Geometry check sheet. Reference: the model listing, model coordinates, mm. Face numbers are marked on the shaded views. A direction names the side the tool comes from. Give positions to 0.01 mm unless a question says otherwise; leave off trailing zeros. Order: outer loops, then holes, each group sorted by start corner. A loop starts at its lowest first (then second) coordinate and runs counter-clockwise, first axis right, second up. Notation, with made-up numbers: M 4,79 L 50,79 A15 cw 50,83 Z; hole C 28.5,73 d4. An arc over 180 degrees is marked long. Answer as CSV lines item,"result".
from build123d import *

# Parameters (mm, degrees)
ESQUISSE1_W             = 18
ESQUISSE1_H             = 34
BOSS_EXTRU_1_DEPTH      = 25
ESQUISSE2_R             = 3
ESQUISSE2_W             = 15
ESQUISSE2_H             = 24
ENL_V_MAT_EXTRU_1_DEPTH = 26
ESQUISSE3_R             = 3
ENL_V_MAT_EXTRU_2_DEPTH = 4
ESQUISSE4_R             = 4
ENL_V_MAT_EXTRU_3_DEPTH = 19


with BuildPart() as part:
    # Esquisse1 → Boss.-Extru.1 (new body)
    with BuildSketch(Plane.XY):
        with Locations((9, -17)):
            Rectangle(ESQUISSE1_W, ESQUISSE1_H)
    extrude(amount=BOSS_EXTRU_1_DEPTH)

    # Esquisse2 → Enlèv. mat.-Extru.1 (cut, through all)
    with BuildSketch(Plane.XY.offset(25)):
        with Locations((8, -29)):
            Circle(ESQUISSE2_R)
        with Locations((7.5, -12)):
            Rectangle(ESQUISSE2_W, ESQUISSE2_H)
    extrude(amount=-ENL_V_MAT_EXTRU_1_DEPTH, mode=Mode.SUBTRACT)

    # Esquisse3 → Enlèv. mat.-Extru.2 (cut)
    with BuildSketch(Plane(origin=(18, 0, 0), x_dir=(0, 0, -1), z_dir=(1, 0, 0))):
        with Locations((-12.5, -29)):
            Circle(ESQUISSE3_R)
    extrude(amount=-ENL_V_MAT_EXTRU_2_DEPTH, mode=Mode.SUBTRACT)

    # Esquisse4 → Enlèv. mat.-Extru.3 (cut, through all)
    with BuildSketch(Plane(origin=(18, 0, 0), x_dir=(0, 0, -1), z_dir=(1, 0, 0))):
        with Locations((-12.5, -6)):
            Circle(ESQUISSE4_R)
    extrude(amount=-ENL_V_MAT_EXTRU_3_DEPTH, mode=Mode.SUBTRACT)


solid = part.part
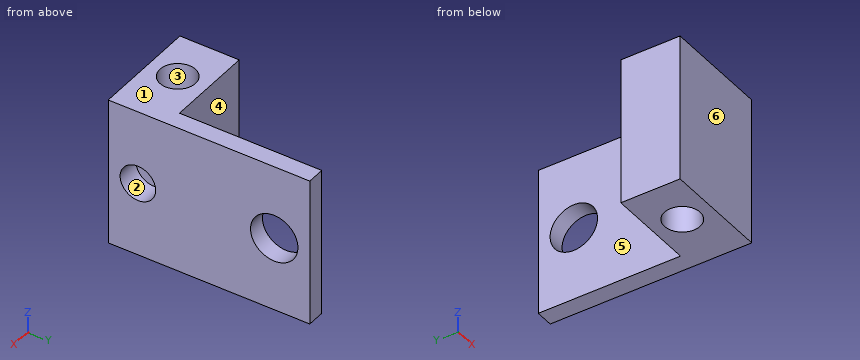
(1) Section check D-D on z = 4.5. Enter the section's corners in (x, y).
The answers:
outline,"M 0,-34 L 18,-34 L 18,0 L 15,0 L 15,-24 L 0,-24 Z; hole C 8,-29 d6"
(2) Section check B-B on y = -6. Enter the section's corners in (x, z), then the cut area to 3 significant figures.
The answers:
outline,"M 15,0 L 18,0 L 18,8.5 L 15,8.5 Z; M 15,16.5 L 18,16.5 L 18,25 L 15,25 Z"
area,"51.0 mm2"
(3) Gauge pin test, flat ends, axial feed: P1, Ø7.5, axis at x = 6, z = 11, coming from the +Y side; P2, Ø10, axis at y = -11.5, z = 17, coming from the -X side. Record the tip position at first contact, or that the pin passes through.
The answers:
P1,"stops at y = -24"
P2,"stops at x = 15"
(4) Section check C-C on x = 8. Enter the section's corners in (y, z), then the cut area to 3 significant figures.
The answers:
outline,"M -34,0 L -32,0 L -32,25 L -34,25 Z; M -26,0 L -24,0 L -24,25 L -26,25 Z"
area,"100 mm2"
(5) Section check A-A on z = 12.5. Enter the section's corners in (x, y), then the cut area to 3 significant figures.
The answers:
outline,"M 0,-34 L 18,-34 L 18,-32 L 14,-32 L 14,-26 L 18,-26 L 18,-10 L 15,-10 L 15,-24 L 0,-24 Z; M 15,-2 L 18,-2 L 18,0 L 15,0 Z; hole C 8,-29 d6"
area,"176 mm2"
(6) Tool access check on the marked faces 5 and 6. Record the directions out of +Z, -Z, +X, -X, +Y, -Y that give a thin tool (end or side, any length) a straight path to the whole face; none if there is none.
The answers:
face 5,"+Z, -Z, -X, +Y"
face 6,"+Z, -Z, +X, -X, -Y"
(7) Material ranges on line 1 (Y direction, x = 17.05, z = 12.5); line 2 (Y direction, x = 8, z = 9.5); line 3 (X direction, y = -22.5, z = 18.75), recorded low to high.
The answers:
line 1,"y = -34 to -32, -26 to -10, -2 to 0"
line 2,"y = -34 to -32, -26 to -24"
line 3,"x = 15 to 18"
(8) Draft check along Y on the marked faces 1, 2, 3 and 4. Enter one of: +Y half, -Y half, draft (parallel to the pull), parting line (faces both ways), or undercut.
The answers:
face 1,"draft"
face 2,"undercut"
face 3,"undercut"
face 4,"+Y half"
